Autodesk Inventor part; units mm, degrees
ref_plane "YZ Plane" through (0, 0, 0) normal (1, 0, 0) x (0, 1, 0)
ref_plane "XZ Plane" through (0, 0, 0) normal (0, 1, 0) x (-1, 0, 0)
ref_plane "XY Plane" through (0, 0, 0) normal (0, 0, 1) x (1, 0, 0)
sketch "草圖1" plane through (0, 0, 0) normal (0, 1, 0) x (-1, 0, 0)
  line L0 (0, 0) -> (42, 0)
  line L1 (42, 0) -> (42, 42)
  line L2 (42, 42) -> (0, 42)
  line L3 (0, 42) -> (0, 0)
  dimension "d0" = 42
  dimension "d1" = 42
extrude "擠出1" add sketch "草圖1" along normal blind 3
sketch "草圖2" plane through (0, 0, 0) normal (0, -1, 0) x (1, 0, 0)
  line L0 (0, 0) -> (-42, 0)
  line L1 (0, 42) -> (0, 0)
  line L2 (-42, 0) -> (0, 0)
  line L3 (0, 0) -> (0, 10)
  line L4 (0, 10) -> (-42, 10)
  line L5 (-42, 10) -> (-42, 0)
  dimension "d4" = 10
extrude "擠出2" add sketch "草圖2" along normal blind 12
sketch "草圖3" plane through (0, 3, 0) normal (0, 1, 0) x (1, 0, 0)
  point P0 (-21, -21)
hole "孔1" at (-21, 3, 21) direction (0, -1, 0) diameter 22 end through all
sketch "草圖4" plane through (0, 3, 0) normal (0, 1, 0) x (1, 0, 0)
  circle A0 centre (-21, -21) radius 11
  point P0 (-36, -6)
  point P1 (-36, -36)
  point P2 (-6, -6)
  point P3 (-6, -36)
  dimension "d15" = 15
  dimension "d16" = 15
  dimension "d17" = 15
  dimension "d18" = 15
hole "孔2" at (-36, 3, 6) at (-36, 3, 36) at (-6, 3, 6) at (-6, 3, 36) direction (0, -1, 0) diameter 3 end through all
fillet "圓角1" radius 3 4 edges at (0, 1.5, 42) (0, -4.5, 0) (-42, 1.5, 42) (-42, -4.5, 0)
sketch "草圖5" plane through (0, 0, 0) normal (0, -1, 0) x (1, 0, 0)
  circle A0 centre (-36, 36) radius 1.5
  point P0 (0, 0)
hole "孔3" at (-36, 0, 36) direction (0, 1, 0) diameter 6 depth 2
sketch "草圖6" plane through (-3, 3, 0) normal (0, 0, -1) x (-1, 0, 0)
  line L0 (0, 0) -> (36, 0)
  line L1 (-3, 0) -> (-3, -15)
  point P0 (-3, -3)
  point P1 (12, -7.5)
  dimension "d35" = 7.5
  dimension "d36" = 15
hole "孔4" at (-15, -4.5, 0) direction (0, 0, 1) diameter 4.917 end through all
sketch "草圖7" plane through (-3, 3, 0) normal (0, 0, -1) x (-1, 0, 0)
  line L0 (39, -15) -> (39, 0)
  point P0 (-3, -3)
  point P1 (29, -7.5)
  dimension "d44" = 10
hole "孔5" at (-32, -4.5, 0) direction (0, 0, 1) diameter 3.242 end through all counterbore diameter 7.5 counterbore depth 2
properties part number "extruder_base"
The listing builds one solid part. Answer for the finished solid, in the listing's coordinates (mm). A direction names the side the tool comes from. Give positions to 0.01 mm unless a question says otherwise; leave off trailing zeros. Order: outer loops, then holes, each group sorted by start corner. A loop starts at its lowest first (then second) coordinate and runs counter-clockwise, first axis right, second up. Notation, with made-up numbers: (60.25, 44.5) - (80.25, 44.5) arc R24 ccw to (80.25, 69.5) - close; hole circle Ø10 at (38, 59.25). An arc over 180 degrees is marked (long way). Use one line per item in the form item = value. Start each with the question number.
(1) Flat-ended cylindrical pins translate along their axes: pin 1 Ø2 at (x, z) = (-34, 25) entering from -Y; pin 2 Ø3 at (x, z) = (-23.5, 31.5) entering from +Y; pin 3 Ø3.5 at (x, y) = (-24, -3) entering from +Z. Find the tip coordinate at first contact, or state that the pin passes through.
(2) Consider line 1 (X direction, y = -4.5, z = 6); line 2 (X direction, y = -4.5, z = 3.25); line 3 (X direction, y = 2.5, z = 36). Determine where each line is inside the solid, lowest interval first. Write a range as from..to.
(3) A cutting plane is placed at B-B, the plane y = -4.5. Write down the section's boundary in (x, z), then the cut area to 3 significant figures.
(4) A cutting plane is placed at A-A, the plane z = 6. Write down the section's boundary in (x, y), then the cut area to 3 significant figures.
(5) A cutting plane is placed at D-D, the plane x = -32.5. Write down the section's boundary in (y, z).
(6) For faces 1 (the cylindrical face through (-38.03, 1.01, 38.21)), 2 (the flat face through (-21, 0, 33)), 3 (the flat face through (-31, -3, 2)), determine the directions among +Z, -Z, +X, -X, +Y, -Y from which every point of the face is accessible in a straight line to the end or side of a thin tool.
(7) A cutting plane is placed at C-C, the plane z = 21. Write down the section's boundary in (x, y), then the cut area to 3 significant figures.
(8) The mould has two halves that part along Y. Classify faces 4 (the cylindrical face through (-30.418, -4.851, 6.056)), 5 (the flat face through (-34.7, 2, 34.7)), 6 (the cylindrical face through (-5.1, 1.5, 34.8)): released by +Y, released by -Y, zero draft, split by the parting line, or undercut.
Ans:
q1.pin_1 = 0
q1.pin_2 = 3
q1.pin_3 = 10
q2.line_1 = -42..-37.5, -34.5..-33.62, -30.38..-17.46, -12.54..-7.5, -4.5..0
q2.line_2 = -42..-33.62, -30.38..-17.46, -12.54..0
q2.line_3 = -42..-37.5, -34.5..-7.5, -4.5..0
q3.outline = (-42, 3) arc R3 ccw to (-39, 0) - (-35.75, 0) - (-35.75, 2) - (-33.62, 2) - (-33.62, 10) - (-42, 10) - close; (-30.38, 2) - (-28.25, 2) - (-28.25, 0) - (-17.46, 0) - (-17.46, 10) - (-30.38, 10) - close; (-12.54, 0) - (-3, 0) arc R3 ccw to (0, 3) - (0, 10) - (-12.54, 10) - close; hole circle Ø3 at (-36, 6); hole circle Ø3 at (-6, 6)
q3.area = 312 mm^2
q4.outline = (-42, -12) - (-37.5, -12) - (-37.5, 3) - (-42, 3) - close; (-34.5, -12) - (-7.5, -12) - (-7.5, 3) - (-34.5, 3) - close; (-4.5, -12) - (0, -12) - (0, 3) - (-4.5, 3) - close; hole circle Ø3.24 at (-32, -4.5); hole circle Ø4.92 at (-15, -4.5)
q4.area = 513 mm^2
q5.outline = (-12, 0) - (-8.22, 0) - (-8.22, 2) - (-6.04, 2) - (-6.04, 10) - (-12, 10) - close; (-2.96, 2) - (-0.78, 2) - (-0.78, 0) - (3, 0) - (3, 42) - (0, 42) - (0, 10) - (-2.96, 10) - close
q6.face_1 = -Y
q6.face_2 = +Z, +X, -X, -Y
q6.face_3 = -Z
q7.outline = (-42, 0) - (-32, 0) - (-32, 3) - (-42, 3) - close; (-10, 0) - (0, 0) - (0, 3) - (-10, 3) - close
q7.area = 60.0 mm^2
q8.face_4 = undercut
q8.face_5 = released by -Y
q8.face_6 = zero draft
